Here's the drawing with two shaded views (mm, measured from the low corner). I have some questions. A direction names the side the tool comes from. Coordinates: 2 decimals unless noted, no trailing zeros. Write each loop counter-clockwise with the first axis right and the second up, starting at its lowest first coordinate (ties: lowest second). Pieces come first, ordered by that corner, then holes.
Item 1: For the marked faces 1, 2, 3, 4 and 5, which set-ups out of +Z, -Z, +X, -X, +Y, -Y let a thin tool reach every point of the face, with its end or its side?
Item 2: I'm going to push flat-ended pins straight in: pin 1 Ø9 at (x, y) = (38.5, 9.5) entering from -Z; pin 2 Ø3.5 at (y, z) = (9, 24.5) entering from +X; pin 3 Ø4 at (y, z) = (9, 7.5) entering from -X. Where does each tip first touch, or does it pass through?
Item 3: If we section it at D-D (y = 15): Please give me the cut outline in (x, z), then the cut area to 3 significant figures.
Item 4: If we section it at A-A (y = 11.75): Please give me the cut outline in (x, z), then the cut area to 4 significant figures.
Item 5: We'd pull the mould along Z, two halves only. Please class the marked faces 6, 7, 8 and 9: +Z half, -Z half, draft (parallel to the pull), parting line (faces both ways), or undercut.
Item 6: If I drill on line 1 (X direction, y = 11.75, z = 25); line 2 (Z direction, x = 34.5, y = 10); line 3 (Y direction, x = 16.5, z = 25), over which ranges is the centre line in solid material (lowest first)?
Item 7: If we section it at B-B (z = 18): Please give me the cut outline in (x, y).
Item 8: If we section it at C-C (x = 31.5): Please give me the cut outline in (y, z), then the cut area to 4 significant figures.
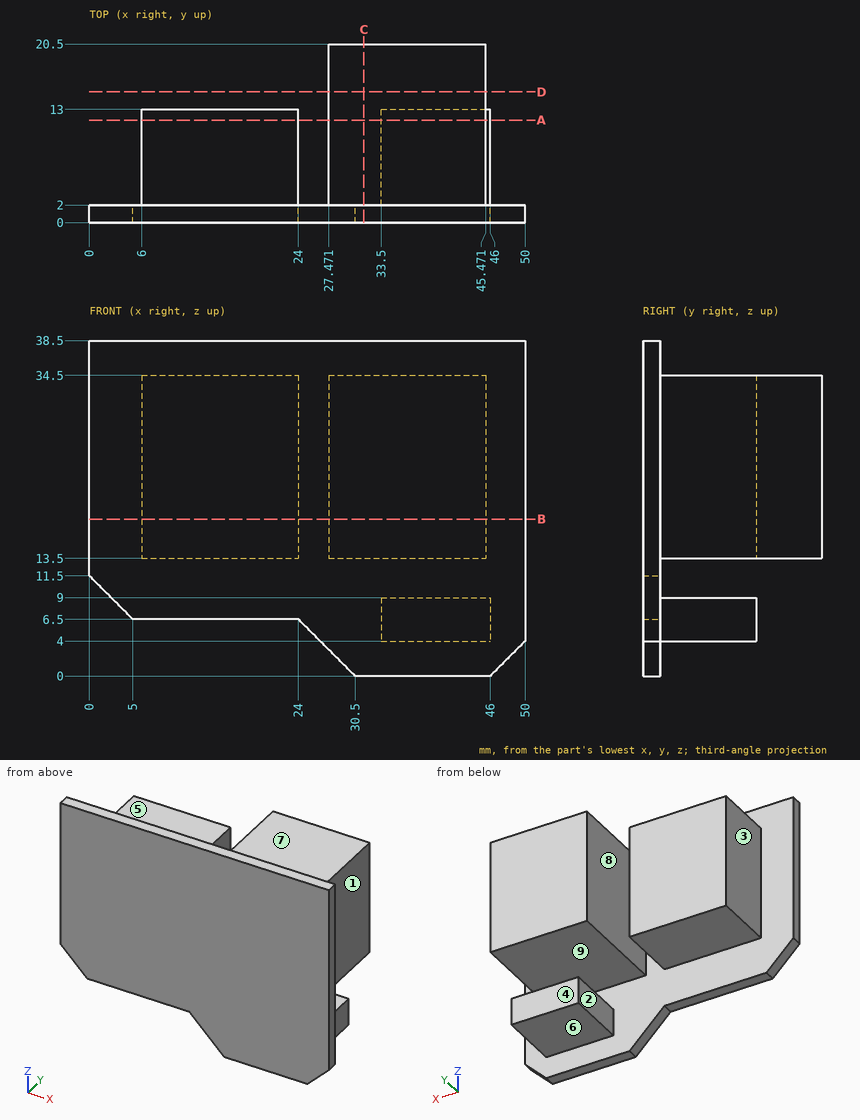
Answer list:
1. face 1: +Z, +X, +Y
1. face 2: -Z, -X, +Y
1. face 3: +Z, -Z, -X, +Y
1. face 4: -Z, +X, -X, +Y
1. face 5: +Z, +X, -X, +Y
2. pin 1: stops at z = 4
2. pin 2: stops at x = 45.47
2. pin 3: stops at x = 33.5
3. outline: (27.47, 13.5) - (45.47, 13.5) - (45.47, 34.5) - (27.47, 34.5) - close
3. area: 378 mm2
4. outline: (6, 13.5) - (24, 13.5) - (24, 34.5) - (6, 34.5) - close; (27.47, 13.5) - (45.47, 13.5) - (45.47, 34.5) - (27.47, 34.5) - close; (33.5, 4) - (46, 4) - (46, 9) - (33.5, 9) - close
4. area: 818.5 mm2
5. face 6: -Z half
5. face 7: +Z half
5. face 8: draft
5. face 9: undercut
6. line 1: x = 6 to 24, 27.47 to 45.47
6. line 2: z = 4 to 9, 13.5 to 34.5
6. line 3: y = 0 to 13
7. outline: (0, 0) - (50, 0) - (50, 2) - (45.47, 2) - (45.47, 20.5) - (27.47, 20.5) - (27.47, 2) - (24, 2) - (24, 13) - (6, 13) - (6, 2) - (0, 2) - close
8. outline: (0, 0) - (2, 0) - (2, 13.5) - (20.5, 13.5) - (20.5, 34.5) - (2, 34.5) - (2, 38.5) - (0, 38.5) - close
8. area: 465.5 mm2
